Can you work these out from the drawing? Everything is in mm from the part's minimum corner. Give positions to 0.01 mm unless a question says otherwise; leave off trailing zeros. Loops run counter-clockwise (first coordinate to the right, second up) from the corner with the lowest first, then second, coordinate; pieces in that order, holes last.
Q1. I need wall thicknesses on line 1 (Y direction, x = 50, z = 5.9); line 2 (Z direction, x = 61, y = 18.5); line 3 (Y direction, x = 47, z = 5.25). Which ranges of each line are inside material? Lowest first, please.
Q2. We'd pull the mould along Y, two halves only. Please class the marked faces 1, 2, 3 and 4: +Y half, -Y half, draft (parallel to the pull), parting line (faces both ways), or undercut.
Q3. If we section it at C-C (z = 7.75): Please give me the cut outline in (x, y), plus the area to 3 significant figures.
Q4. If we section it at A-A (x = 50): Please give me the cut outline in (y, z).
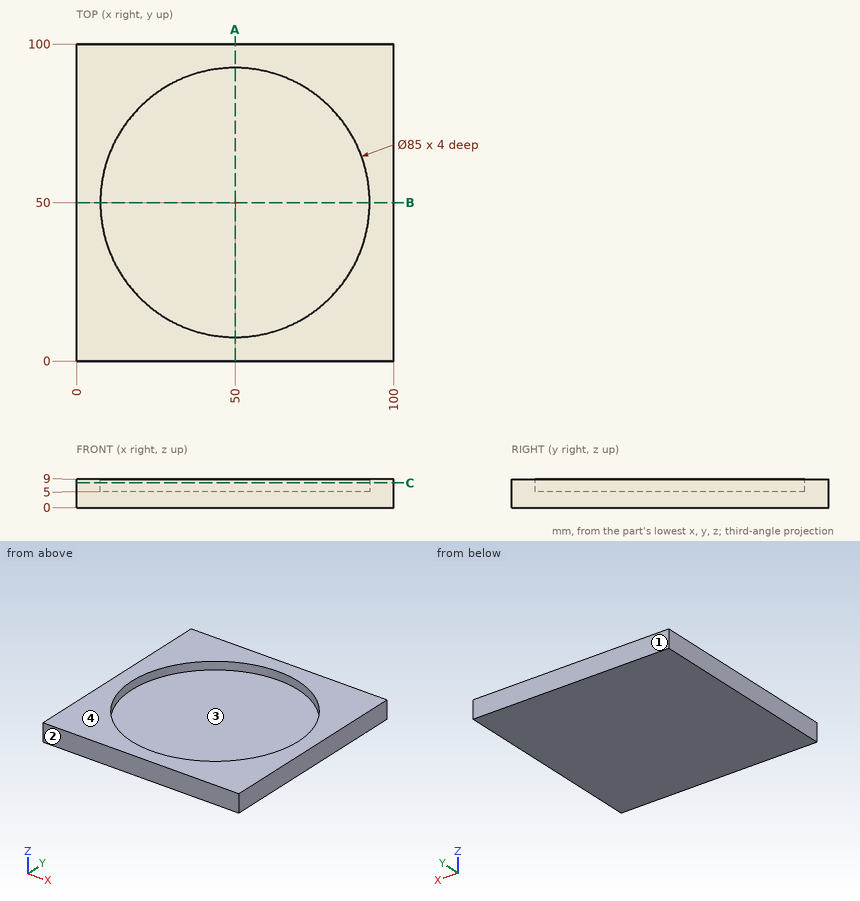
Check sheet entries:
1. line 1: y = 0 to 7.5, 92.5 to 100
1. line 2: z = 0 to 5
1. line 3: y = 0 to 7.61, 92.39 to 100
2. face 1: +Y half
2. face 2: -Y half
2. face 3: undercut
2. face 4: draft
3. outline: (0, 0) - (100, 0) - (100, 100) - (0, 100) - close; hole circle Ø85 at (50, 50)
3. area: 4,330 mm2
4. outline: (0, 0) - (100, 0) - (100, 9) - (92.5, 9) - (92.5, 5) - (7.5, 5) - (7.5, 9) - (0, 9) - close
